Geometry check sheet. Reference: the model listing, model coordinates, mm. Coordinates: 2 decimals unless noted, no trailing zeros. Write each loop counter-clockwise with the first axis right and the second up, starting at its lowest first coordinate (ties: lowest second). Pieces come first, ordered by that corner, then holes. Notation, with made-up numbers: M 39,15.25 L 94,15.25 A13 ccw 94,37.25 Z; hole C 7,36 d7. An arc over 180 degrees is marked long. Write each question's results on one line, items separated by ' | '.
```python
from build123d import *


with BuildPart() as f3:
    # F0 (on Front) → F3 section 0
    with BuildSketch(Plane.XZ, mode=Mode.PRIVATE) as f3_s0:
        Polygon((-26.928486, 42.739754), (-50.204922, 5.594263), (-35.676027, -35.763822), (5.717643, -50.19102), (42.805812, -26.823356), (47.660331, 16.742842), (16.625649, 47.701339), align=None)
    loft([f3_s0.sketch, Vertex(0, -25, 0)])


solid = f3.part
```
Q1. Sectioned sample at C-C on z = -15. Record the cut outline in (x, y), and give its area (3 significant figures).
Geometry check:
outline: M -42.97,0 L -14.96,-14.51 L 1.71,-17.53 L 23.94,-11.02 L 44.12,0 Z | area: 899 mm2
Q2. Sectioned sample at D-D on y = -10.5. Record the cut outline in (x, z).
Geometry check:
outline: M -29.12,3.24 L -20.69,-20.74 L 3.32,-29.11 L 24.83,-15.56 L 27.64,9.71 L 9.64,27.67 L -15.62,24.79 Z
Q3. Depth check by flat-ended pin: P1, Ø5, axis at x = 36.5, y = -10, coming from the -Z side; P2, Ø5, axis at x = 31.5, z = 5.5, coming from the +Y side; P3, Ø1.5, axis at x = 28, z = -3.5, coming from the -Y side; P4, Ø3, axis at x = -5, y = -20.5, coming from the -Z side. Enter the tip coordinate at first touch or a pass-through.
Geometry check:
P1: passes through | P2: stops at y = 0 | P3: stops at y = -9.91 | P4: stops at z = -9.87
Q4. Mould release check, pull along X, two halves, no side actions. Record for faces 1 (the flat face through (27.29, -9.9, -3.35)), 2 (the flat face through (-3, 0, -2)), 3 (the flat face through (-26.04, -9.9, -8.82)): pulls with the +X half, pulls with the -X half, needs draft (parallel to the pull), parting line crosses it, or undercut.
Geometry check:
face 1: pulls with the +X half | face 2: needs draft | face 3: pulls with the -X half
Q5. Sectioned sample at B-B on x = 2. Record the cut outline in (y, z), and give its area (3 significant figures).
Geometry check:
outline: M -23.95,0.7 L -23.83,-1.25 L -16.26,-17.56 L 0,-48.9 L 0,46.04 L -21.99,5.74 Z | area: 1,190 mm2
Q6. Sectioned sample at A-A on y = -19.5. Record the cut outline in (x, z).
Geometry check:
outline: M -11.05,1.23 L -7.85,-7.87 L 1.26,-11.04 L 9.42,-5.9 L 10.49,3.68 L 3.66,10.49 L -5.92,9.4 Z
Q7. Scan lines: probe 1 along Y at (x, z) = (-16, 14); probe 2 along Z at (x, y) = (-3, -1.25); probe 3 along Y at (x, z) = (16.5, 25.5). Record each from-to range of solid material in increasing order.
Geometry check:
probe 1: y = -13.47 to 0 | probe 2: z = -44.74 to 43.18 | probe 3: y = -8.68 to 0
